Geometry check sheet. Reference: the model listing, model coordinates, mm. A direction names the side the tool comes from. Round coordinates to 2 decimals unless told otherwise and drop trailing zeros. Order: outer loops, then holes, each group sorted by start corner. A loop starts at its lowest first (then second) coordinate and runs counter-clockwise, first axis right, second up. Notation, with made-up numbers: (33, 83.25) - (65, 83.25) arc R9 ccw to (65, 99.25) - close; hole circle Ø1 at (-20.5, -4). An arc over 180 degrees is marked (long way). Use a Markdown table: item, result. Add a question column.
(1) Section check C-C on x = 19.5. Record the boundary of the cut face in (y, z).
(2) Mould release check, pull along Z, two halves, no side actions. Record for faces 1 (the face through (0, 10.16, 54)), 2 (the face through (-1, -23, -60)), 3 (the face through (57.5, -22, -1)), 4 (the face through (1, 0, 47)): released by +Z, released by -Z, zero draft, split by the parting line, or undercut.
(3) Section check B-B on z = -51. Record the boundary of the cut face in (x, y), then the cut area to 3 significant figures.
(4) Section check A-A on y = -53. Record the boundary of the cut face in (x, z).
(5) Gauge pin test, flat ends, axial feed: P1, Ø3, axis at x = 3.5, y = 12, coming from the +Z side; P2, Ø4, axis at x = -33, z = 55.5, coming from the +Y side; P3, Ø3, axis at x = -7, z = 12, coming from the +Y side. Record the tip position at first contact, or that the pin passes through.
(6) Thickness scan on line 1 along Z through (x, y) = (12, -15.5); line 2 along X through (y, z) = (-23, 41); line 3 along Z through (x, y) = (-50.5, 3.5). Record the ranges inside material, lowest first. Write a range as [from, to].
(7) Section check D-D on z = 22. Record the boundary of the cut face in (x, y).
(8) Access from +Z, -Z, +X, -X, +Y, -Y to the whole of each face (thin tool, end or side, straight path). Record for faces 5 (the face through (38, 10.16, 54)), 6 (the face through (1, -24, 60)), 7 (the face through (1, 6, 39.68)), 8 (the face through (1, 0, -38)).
```python
from build123d import *

# Parameters (mm, degrees)
F0_W     = 125
F0_H     = 120
F1_DEPTH = 60
F2_W     = 125
F2_H     = 20.32
F2_H_2   = 38.1
F3_DEPTH = 12.7
F4_W     = 115
F4_H     = 110
F5_DEPTH = 55
F6_W     = 25.4
F6_H     = 12.7
F7_DEPTH = 2.54
F8_W     = 5
F8_H     = 61.58
F9_DEPTH = 12.7


with BuildPart() as f1:
    # F0 (on Front) → F1 (new body)
    with BuildSketch(Plane.XZ):
        Rectangle(F0_W, F0_H)
    extrude(amount=F1_DEPTH)

    # F2 (on face) → F3 (join)
    with BuildSketch(Plane(origin=(0, 0, 0), x_dir=(-1, 0, 0), z_dir=(0, 1, 0))):
        with Locations((0, 49.84)):
            Rectangle(F2_W, F2_H)
        with Locations((0, -40.95)):
            Rectangle(F2_W, F2_H_2)
    extrude(amount=F3_DEPTH)

    # F4 (on face) → F5 (cut)
    with BuildSketch(Plane(origin=(0, 0, 0), x_dir=(-1, 0, 0), z_dir=(0, 1, 0))):
        Rectangle(F4_W, F4_H)
    extrude(amount=-F5_DEPTH, mode=Mode.SUBTRACT)

    # F6 (on face) → F7 (cut)
    with BuildSketch(Plane(origin=(0, 12.7, 0), x_dir=(-1, 0, 0), z_dir=(0, 1, 0))):
        with Locations((-37.592, 53.65)):
            Rectangle(F6_W, F6_H)
        Polygon((12.7, 60), (0, 60), (-12.7, 60), (-12.7, 47.3), (0, 47.3), (12.7, 47.3), align=None)
        with Locations((37.592, 53.65)):
            Rectangle(F6_W, F6_H)
    extrude(amount=-F7_DEPTH, mode=Mode.SUBTRACT)

    # F8 (on face) → F9 (join)
    with BuildSketch(Plane(origin=(0, 0, 0), x_dir=(-1, 0, 0), z_dir=(0, 1, 0))):
        with Locations((60, 8.89)):
            Rectangle(F8_W, F8_H)
        with Locations((-60, 8.89)):
            Rectangle(F8_W, F8_H)
    extrude(amount=F9_DEPTH)


solid = f1.part
```
Check sheet entries:
| question | item | result |
|---|---|---|
| 1 | outline | (-60, -60) - (12.7, -60) - (12.7, -21.9) - (0, -21.9) - (0, -55) - (-55, -55) - (-55, 55) - (0, 55) - (0, 39.68) - (12.7, 39.68) - (12.7, 60) - (-60, 60) - close |
| 2 | face 1 | zero draft |
| 2 | face 2 | released by -Z |
| 2 | face 3 | undercut |
| 2 | face 4 | undercut |
| 3 | outline | (-62.5, -60) - (62.5, -60) - (62.5, 12.7) - (-62.5, 12.7) - close; hole (-57.5, -55) - (57.5, -55) - (57.5, 0) - (-57.5, 0) - close |
| 3 | area | 2,760 mm2 |
| 4 | outline | (-62.5, -60) - (62.5, -60) - (62.5, 60) - (-62.5, 60) - close; hole (-57.5, -55) - (57.5, -55) - (57.5, 55) - (-57.5, 55) - close |
| 5 | P1 | stops at z = 47.3 |
| 5 | P2 | stops at y = 10.16 |
| 5 | P3 | stops at y = -55 |
| 6 | line 1 | z = [-60, -55], [55, 60] |
| 6 | line 2 | x = [-62.5, -57.5], [57.5, 62.5] |
| 6 | line 3 | z = [-60, -21.9], [39.68, 60] |
| 7 | outline | (-62.5, -60) - (62.5, -60) - (62.5, 12.7) - (57.5, 12.7) - (57.5, -55) - (-57.5, -55) - (-57.5, 12.7) - (-62.5, 12.7) - close |
| 8 | face 5 | +Z, +Y |
| 8 | face 6 | +Z, +X, -X, +Y, -Y |
| 8 | face 7 | +Y |
| 8 | face 8 | none |
